Read the model definition and answer for the solid it produces. Units are mm, in the model's axes. A direction names the side the tool comes from. Coordinates: 2 decimals unless noted, no trailing zeros. Order: outer loops, then holes, each group sorted by start corner. A loop starts at its lowest first (then second) coordinate and runs counter-clockwise, first axis right, second up. Notation, with made-up numbers: (78, 7.25) - (123, 7.25) arc R4 ccw to (123, 12.25) - close; hole circle Ø9 at (-4.5, -17). An arc over 180 degrees is marked (long way). Answer as a JSON object with one key per item and string values. Group by question number.
from build123d import *

# Parameters (mm, degrees)
F1_DEPTH  = 41.5
F2_DEPTH  = 35.5
F3_DEPTH  = 6
F5_DEPTH  = 50
F6_R      = 2.5
F7_DEPTH  = 5
F8_DEPTH  = 19.5
F9_DEPTH  = 5
F10_DEPTH = 50
F11_R     = 2


with BuildPart() as f1:
    # F0 (on Top) → F1 (new body)
    with BuildSketch(Plane.XY):
        with BuildLine():
            Line((30, 19), (30, -19))
            Line((30, -19), (33, -19))
            Line((33, -19), (33, 19))
            Line((33, 19), (33, 20))
            ThreePointArc((33, 20), (31.5355339059, 23.5355339059), (28, 25))
            Line((28, 25), (-28, 25))
            ThreePointArc((-28, 25), (-31.5355339059, 23.5355339059), (-33, 20))
            Line((-33, 20), (-33, 19))
            Line((-33, 19), (-33, -19))
            Line((-33, -19), (-30, -19))
            Line((-30, -19), (-30, 19))
            Line((-30, 19), (-10, 19))
            Line((-10, 19), (-6, 23))
            Line((-6, 23), (6, 23))
            Line((6, 23), (10, 19))
            Line((10, 19), (30, 19))
        make_face()
    extrude(amount=F1_DEPTH)

    # F0 (on Top) → F2 (join)
    with BuildSketch(Plane.XY):
        Polygon((-30, -19), (30, -19), (30, 19), (10, 19), (-10, 19), (-30, 19), align=None)
        Polygon((-10, 19), (10, 19), (6, 23), (-6, 23), align=None)
    extrude(amount=F2_DEPTH)

    # F0 (on Top) → F3 (cut)
    with BuildSketch(Plane.XY):
        Polygon((-30, -19), (30, -19), (30, 19), (10, 19), (-10, 19), (-30, 19), align=None)
        Polygon((-10, 19), (10, 19), (6, 23), (-6, 23), align=None)
    extrude(amount=F3_DEPTH, mode=Mode.SUBTRACT)

    # F4 (on face) → F5 (cut)
    with BuildSketch(Plane.XY.offset(35.5)):
        Polygon((6, 13), (-6, 13), (-10, 17), (-28, 17), (-28, 12), (-30, 12), (-30, -14), (-28, -14), (-28, -19), (28, -19), (28, -14), (30, -14), (30, 12), (28, 12), (28, 17), (10, 17), align=None)
    extrude(amount=-F5_DEPTH, mode=Mode.SUBTRACT)

    # F6 (on face) → F7 (cut)
    with BuildSketch(Plane.XY.offset(35.5)):
        Polygon((-6, 23), (-10, 19), (-10, 17), (-6, 13), (6, 13), (10, 17), (10, 19), (6, 23), align=None)
        with Locations((0, 18)):
            Circle(F6_R, mode=Mode.SUBTRACT)
    extrude(amount=-F7_DEPTH, mode=Mode.SUBTRACT)

    # F8 (cut): a face of the model
    f8_faces = [f1.faces().sort_by_distance(p)[0] for p in [
        (-7.841886117, 20.841886117, 30.5),
    ]]
    extrude(f8_faces, amount=-F8_DEPTH, mode=Mode.SUBTRACT)

    # F6 (on face) → F9 (join)
    with BuildSketch(Plane.XY.offset(35.5)):
        Polygon((-6, 23), (-10, 19), (-10, 17), (-6, 13), (6, 13), (10, 17), (10, 19), (6, 23), align=None)
        with Locations((0, 18)):
            Circle(F6_R, mode=Mode.SUBTRACT)
    extrude(amount=-F9_DEPTH)

    # F6 (on face) → F10 (cut)
    with BuildSketch(Plane.XY.offset(35.5)):
        with Locations((0, 18)):
            Circle(F6_R)
    extrude(amount=-F10_DEPTH, mode=Mode.SUBTRACT)

    # F11
    f11_edges = [f1.edges().sort_by_distance(p)[0] for p in [
        (-33, -19, 20.75),
        (33, -19, 20.75),
    ]]
    fillet(f11_edges, radius=F11_R)


solid = f1.part
1. A cutting plane is placed at C-C on z = 22. Write down the section's boundary in (x, y), and give its area (3 significant figures).
2. Straight lines are drawn through the part: L1, parallel to Y at x = 0, z = 32; L2, parallel to X at y = 12.5, z = 14; L3, parallel to X at y = 8, z = 32. For each, find the intervals that lie inside material, in ascending order.
3. Given pin 1 (9 mm diameter, centred on x = 20, z = 18, fed in from -Y); pin 2 (0.6 mm diameter, centred on x = -29.5, z = 22, fed in from +Y); pin 3 (9.5 mm diameter, centred on x = -0.5, z = 18.5, fed in from -Y), each flat-ended and moving along its own axis, determine where each tip first touches the part or whether it passes through.
4. For faces 4 (the flat face through (-29, 12, 21)), 5 (the flat face through (28, -17, 21)), 6 (the flat face through (-8, 21, 38)), 7 (the flat face through (-8, 21, 3)), 8 (the flat face through (-2.4, 19.2, 30.5)), determine the directions among +Z, -Z, +X, -X, +Y, -Y from which every point of the face is accessible in a straight line to the end or side of a thin tool.
5. For a pull along Z with two mould halves and no side action, classify faces 1 (the flat face through (8, 21, 21)), 2 (the flat face through (8, 21, 3)), 3 (the flat face through (-29, -16, 35.5)) as pulls with the +Z half, pulls with the -Z half, needs draft (parallel to the pull), parting line crosses it, or undercut.
6. A cutting plane is placed at D-D on x = 14. Write down the section's boundary in (y, z), and give its area (3 significant figures).
7. A cutting plane is placed at B-B on x = 0. Write down the section's boundary in (y, z), and give its area (3 significant figures).
8. A cutting plane is placed at A-A on y = 9. Write down the section's boundary in (x, z).
Derived:
{
 "1": {"outline": "(-33, -17) arc R2 ccw to (-31, -19) - (-28, -19) - (-28, -14) - (-30, -14) - (-30, 12) - (-28, 12) - (-28, 17) - (-10, 17) - (-10, 19) - (-6, 23) - (6, 23) - (10, 19) - (10, 17) - (28, 17) - (28, 12) - (30, 12) - (30, -14) - (28, -14) - (28, -19) - (31, -19) arc R2 ccw to (33, -17) - (33, 20) arc R5 ccw to (28, 25) - (-28, 25) arc R5 ccw to (-33, 20) - close", "area": "668 mm2"},
 "2": {"L1": "y = 13 to 15.5, 20.5 to 25", "L2": "x = -33 to -28, 28 to 33", "L3": "x = -33 to -30, 30 to 33"},
 "3": {"pin 1": "stops at y = 17", "pin 2": "stops at y = 24.85", "pin 3": "stops at y = 23"},
 "4": {"face 4": "+Z, -Z", "face 5": "+Z, -Z, -Y", "face 6": "+Z, -Y", "face 7": "-Z, -Y", "face 8": "-Y"},
 "5": {"face 1": "undercut", "face 2": "needs draft", "face 3": "pulls with the +Z half"},
 "6": {"outline": "(17, 6) - (19, 6) - (19, 0) - (25, 0) - (25, 41.5) - (19, 41.5) - (19, 35.5) - (17, 35.5) - close", "area": "308 mm2"},
 "7": {"outline": "(13, 6) - (15.5, 6) - (15.5, 11) - (13, 11) - close; (13, 30.5) - (15.5, 30.5) - (15.5, 35.5) - (13, 35.5) - close; (20.5, 6) - (23, 6) - (23, 0) - (25, 0) - (25, 41.5) - (23, 41.5) - (23, 35.5) - (20.5, 35.5) - (20.5, 30.5) - (23, 30.5) - (23, 11) - (20.5, 11) - close", "area": "133 mm2"},
 "8": {"outline": "(-33, 0) - (-30, 0) - (-30, 41.5) - (-33, 41.5) - close; (30, 0) - (33, 0) - (33, 41.5) - (30, 41.5) - close"}
}
